Autodesk Inventor part; units mm, degrees
ref_plane "to_screw1_XY" through (0, 5, 0) normal (0, 1, 0) x (1, 0, 0)
ref_plane "to_screw1_YZ" through (0, 5, 0) normal (1, 0, 0) x (0, 0, -1)
ref_plane "to_screw1_ZX" through (0, 5, 0) normal (0, 0, -1) x (0, 1, 0)
sketch "Sketch_1" plane through (0, 0, 0) normal (0, 0, 1) x (1, 0, 0)
  line L0 (2, 0) -> (-2, 0)
  line L1 (-2.5, 5.2) -> (-2.3, 5)
  line L2 (-2.3, 5) -> (2.3, 5)
  line L3 (2.3, 5) -> (2.5, 5.2)
  line L4 (2.5, 5.2) -> (2.5, 7.8)
  line L5 (2.5, 7.8) -> (2.3, 8)
  line L6 (2.3, 8) -> (-2.3, 8)
  line L7 (-2.3, 8) -> (-2.5, 7.8)
  line L8 (-2.5, 7.8) -> (-2.5, 5.2)
revolve "Revolution1" add sketch "Sketch_1" angle 360 about axis through (2, 0, 0) along (1, 0, 0)
sketch "Sketch_2" plane through (0, 0, 0) normal (0, 1, 0) x (-1, 0, 0)
  line L0 (0, 8) -> (0, 5)
  line L1 (0, 4) -> (-1.2295, 4)
  line L2 (-1.2295, 4) -> (-1.2295, 7.459)
  line L3 (-1.2295, 7.459) -> (-1.6074, 7.8369)
  line L4 (-1.6074, 7.8369) -> (-1.6074, 8.25)
  line L5 (-1.6074, 8.25) -> (0, 8.25)
  line L6 (0, 8.25) -> (0, 4)
revolve "Revolution2" cut sketch "Sketch_2" angle 360 about axis through (0, 0, 8) along (0, 0, 1)
thread "Thread1"
sketch "Sketch_6" plane through (0, 0, 0) normal (0, 0, 1) x (1, 0, 0)
  line L0 (0, 8) -> (0, 5)
  line L1 (0, 4) -> (-1.2295, 4)
  line L2 (-1.2295, 4) -> (-1.2295, 7.459)
  line L3 (-1.2295, 7.459) -> (-1.6074, 7.8369)
  line L4 (-1.6074, 7.8369) -> (-1.6074, 8.25)
  line L5 (-1.6074, 8.25) -> (0, 8.25)
  line L6 (0, 8.25) -> (0, 4)
revolve "Revolution3" cut sketch "Sketch_6" angle 360 about axis through (0, 8, 0) along (0, 1, 0)
thread "Thread2"
ref_plane "to_screw1_XY" through (0, 5, 0) normal (0, 1, 0) x (1, 0, 0)
ref_plane "to_screw1_YZ" through (0, 5, 0) normal (1, 0, 0) x (0, 0, -1)
ref_plane "to_screw1_ZX" through (0, 5, 0) normal (0, 0, -1) x (0, 1, 0)
ref_plane "to_screw2_XY" through (0, 0, 5) normal (0, 0, 1) x (1, 0, 0)
ref_plane "to_screw2_YZ" through (0, 0, 5) normal (1, 0, 0) x (0, 1, 0)
ref_plane "to_screw2_ZX" through (0, 0, 5) normal (0, 1, 0) x (0, 0, 1)
properties part number "SCCJ10-5_b"
The model under review builds one solid part; all positions refer to its coordinate system, in mm. A direction names the side the tool comes from. Give positions to 0.01 mm unless a question says otherwise; leave off trailing zeros. Loops run counter-clockwise (first coordinate to the right, second up) from the corner with the lowest first, then second, coordinate; pieces in that order, holes last. Notation, with made-up numbers: (-17.75, -33.5) - (38.25, -33.5) arc R14 cw to (38.25, -10.5) - close; hole circle Ø11 at (30, 78). An arc over 180 degrees is marked (long way). Answer as a JSON object with one key per item and string values.
Q1. Mouldability with a two-part tool opening along Y and no side actions: class faces 4 (the flat face through (2.5, 2, -5)), 5 (the cylindrical face through (0.03, -1.08, -4.88)), 6 (the cylindrical face through (-0.03, 3.69, 7.1)) as +Y half, -Y half, draft (parallel to the pull), parting line (faces both ways), or undercut.
Worked out:
{"face 4": "draft", "face 5": "undercut", "face 6": "parting line"}
Q2. For faces 1 (the flat face through (-2.5, 2, -5)), 2 (the cylindrical face through (0.976, 6.171, -0.748)), 3 (the cylindrical face through (-0.976, -0.748, 6.171)), list the 3-axis set-ups (+Z, -Z, +X, -X, +Y, -Y) from which the entire face can be reached by the end or side of a thin tool; tool diameter is ignored.
Worked out:
{"face 1": "+Z, -Z, -X, +Y, -Y", "face 2": "+Y", "face 3": "+Z"}
Q3. Add section A-A on z = 0. State the section outline as (x, y) points, plus the area to 3 significant figures.
Worked out:
{"outline": "(-2.5, -7.8) - (-2.3, -8) - (2.3, -8) - (2.5, -7.8) - (2.5, -5.2) - (2.3, -5) - (-2.3, -5) - (-2.5, -5.2) - close; (-2.5, 5.2) - (-2.3, 5) - (-1.23, 5) - (-1.23, 7.46) - (-1.61, 7.84) - (-1.61, 8) - (-2.3, 8) - (-2.5, 7.8) - close; (1.23, 5) - (2.3, 5) - (2.5, 5.2) - (2.5, 7.8) - (2.3, 8) - (1.61, 8) - (1.61, 7.84) - (1.23, 7.46) - close", "area": "22.2 mm^2"}
Q4. To check wall thickness, follow line 1 along X through (y, z) = (5.8, 0); line 2 along Z through (x, y) = (-2.05, 0); line 3 along Y through (x, z) = (0.3, 5.75). State the ranges of each line that lie inside material, in increasing order.
Worked out:
{"line 1": "x = -2.5 to -1.23, 1.23 to 2.5", "line 2": "z = -8 to -5, 5 to 8", "line 3": "y = -5.56 to -1.19, 1.19 to 5.56"}
Q5. Insertion check: pin 1 (3 mm diameter, centred on x = 0, z = 0, fed in from +Y); pin 2 (2 mm diameter, centred on x = -1.5, z = 1, fed in from +Y). Each pin has a flat end and moves straight along its axis. Give the tip position at first contact, or say it passes through.
Worked out:
{"pin 1": "stops at y = 7.73", "pin 2": "stops at y = 8"}
